Design review of the part shown in the three views and the two pictorial views. Dimensions are in mm from the part's minimum x, y and z. A direction names the side the tool comes from. Coordinates: 2 decimals unless noted, no trailing zeros. Loops run counter-clockwise (first coordinate to the right, second up) from the corner with the lowest first, then second, coordinate; pieces in that order, holes last. Notation, with made-up numbers: (3, -9) -> (24, -9) arc R21 ccw to (24, 6) -> close; hole circle Ø10 at (87.5, -28). An arc over 180 degrees is marked (long way). One line per item, written item: value.
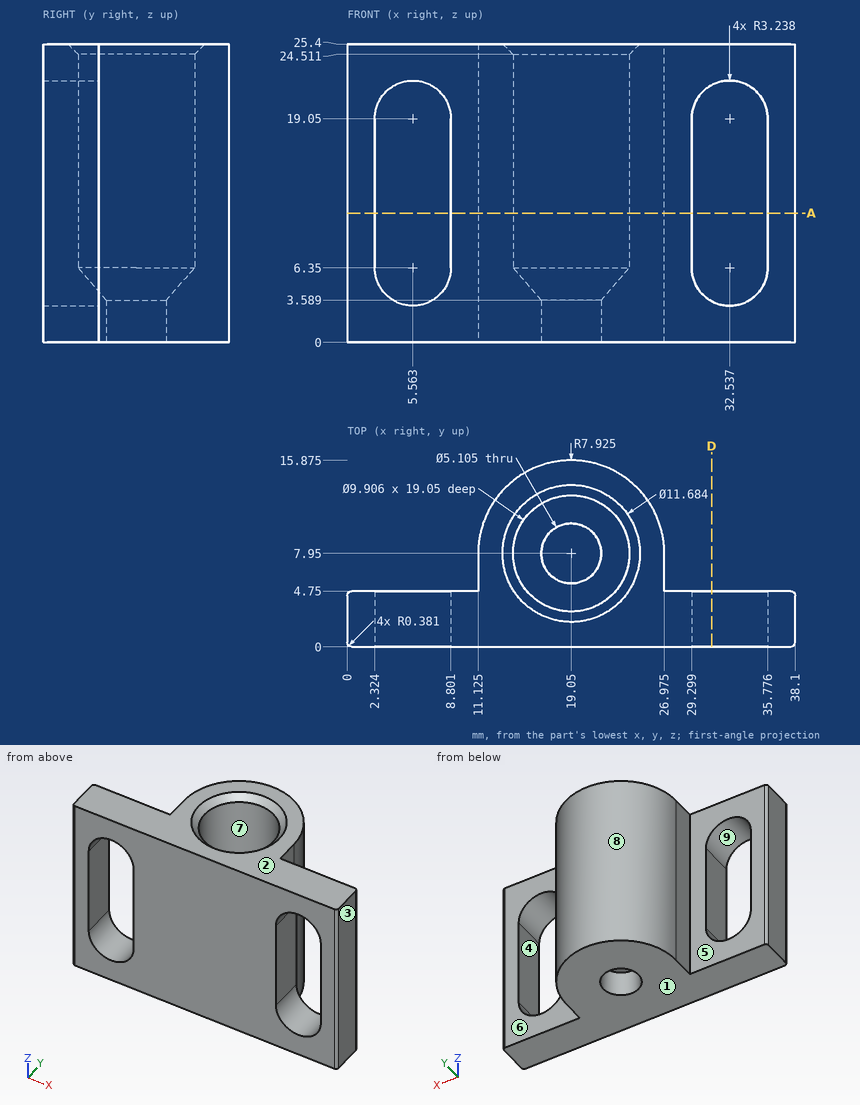
1. Take a section at D-D, the plane x = 31. Give the boundary of the cut face in (y, z).
Return value:
outline: (0, 0) -> (4.75, 0) -> (4.75, 3.5) -> (0, 3.5) -> close; (0, 21.9) -> (4.75, 21.9) -> (4.75, 25.4) -> (0, 25.4) -> close
2. Take a section at A-A, the plane z = 11. Give the number of separate pieces and of enclosed holes in the cut face.
Return value:
separate pieces: 3
enclosed holes: 1
3. For the marked faces 5, 6, 7, 8 and 9, list the 3-axis set-ups (+Z, -Z, +X, -X, +Y, -Y) from which the entire face can be reached by the end or side of a thin tool; tool diameter is ignored.
Return value:
face 5: +Z, -Z, -X, +Y
face 6: +Z, -Z, +X, +Y
face 7: +Z
face 8: +Z, -Z, +Y
face 9: +Y, -Y
4. To check wall thickness, follow probe 1 along Y at (x, z) = (19.05, 14.25) (1 decimal); probe 2 along X at (y, z) = (2.5, 11.5) (1 decimal); probe 3 along X at (y, z) = (4.5, 15) (1 decimal). State the ranges of each line that lie inside material, in increasing order. Write a range as from..to.
Return value:
probe 1: y = 0..3, 12.9..15.9
probe 2: x = 0..2.3, 8.8..29.3, 35.8..38.1
probe 3: x = 0..2.3, 8.8..15.5, 22.6..29.3, 35.8..38.1
5. The part is to be moulded in two halves that separate along Z. For the marked faces 1, 2, 3 and 4, say which applies: pulls with the +Z half, pulls with the -Z half, needs draft (parallel to the pull), parting line crosses it, or undercut.
Return value:
face 1: pulls with the -Z half
face 2: pulls with the +Z half
face 3: needs draft
face 4: undercut
6. Insertion check: pin 1 Ø12 at (x, z) = (34, 9.5) entering from +Y; pin 2 Ø9 at (x, y) = (19.05, 7.95) entering from +Z; pin 3 Ø1.4 at (y, z) = (3, 11.5) entering from -X; pin 4 Ø1 at (y, z) = (7, 8.5) entering from +X (1 decimal). Each pin has a flat end and moves straight along its axis. Give the tip position at first contact, or say it passes through.
Return value:
pin 1: stops at y = 4.75
pin 2: stops at z = 5.83
pin 3: stops at x = 0
pin 4: stops at x = 27
